Study the drawing (mm; zero at the part's minimum x, y, z) and answer. A direction names the side the tool comes from. Give positions to 0.01 mm unless a question says otherwise; leave off trailing zeros. Order: outer loops, then holes, each group sorted by start corner. A loop starts at its lowest first (then second) coordinate and runs counter-clockwise, first axis right, second up. Notation, with made-up numbers: (-32.75, 1.5) - (-10.75, 1.5) arc R29 cw to (-10.75, 37.5) - close; hole circle Ø11 at (27.5, -34.5). An arc over 180 degrees is marked (long way). Write each question's results on one line, items separated by ' | '. Start each with the question number.
1. Which of the six approach directions +Z, -Z, +X, -X, +Y, -Y give full straight-line access (tool end or side, diameter ignored) to the marked faces 4, 5 and 6?
2. Flat-ended cylindrical pins translate along their axes: pin 1 (2 mm diameter, centred on x = 10.5, y = 4, fed in from -Z); pin 2 (2 mm diameter, centred on x = 6.5, y = 7.5, fed in from +Z); pin 3 (1.5 mm diameter, centred on x = 4, z = 6.5, fed in from -Y). Find the tip coordinate at first contact, or state that the pin passes through.
3. Determine the mould class of the marked faces 1, 2 and 3 for opening direction X: released by +X, released by -X, zero draft, split by the parting line, or undercut.
4. Find the intervals of material crossed by L1, parallel to X at y = 1.5, z = 12; L2, parallel to Z at x = 1.5, y = 0.5; L3, parallel to Y at x = 3, z = 17.25, in increasing order.
5. Section B-B (z = 9.25) is taken. Give the vertices of the cut face in (x, y), and give its area (3 significant figures).
6. Section A-A (y = 3.75) is taken. Give the vertices of the cut face in (x, z), and give its area (3 significant figures).
7. Section C-C (x = 3.5) is taken. Give the vertices of the cut face in (y, z).
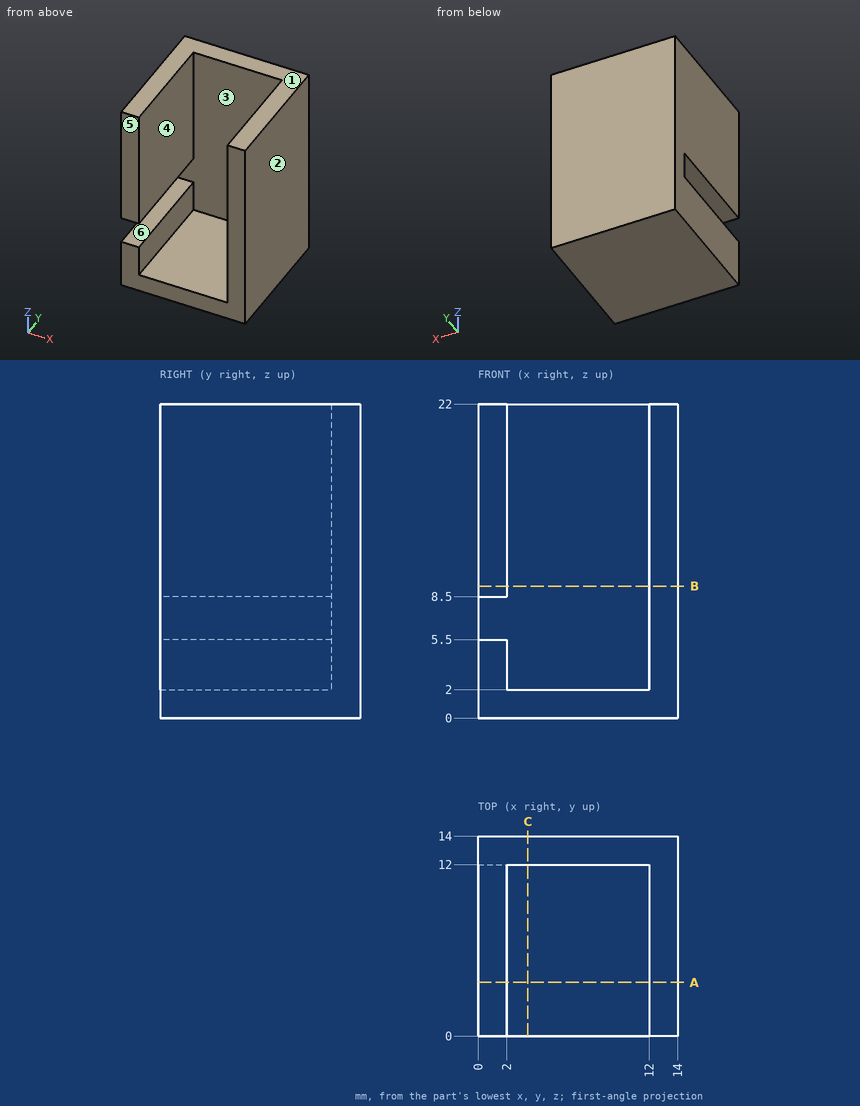
Reported:
1) face 4: +Z, -Y | face 5: +Z, -Z, +X, -X, -Y | face 6: -X, -Y
2) pin 1: z = 0 | pin 2: z = 2 | pin 3: y = 12
3) face 1: zero draft | face 2: released by +X | face 3: undercut
4) L1: 0 to 2, 12 to 14 | L2: 0 to 5.5, 8.5 to 22 | L3: 12 to 14
5) outline: (0, 0) - (2, 0) - (2, 12) - (12, 12) - (12, 0) - (14, 0) - (14, 14) - (0, 14) - close | area: 76.0 mm²
6) outline: (0, 0) - (14, 0) - (14, 22) - (12, 22) - (12, 2) - (2, 2) - (2, 5.5) - (0, 5.5) - close; (0, 8.5) - (2, 8.5) - (2, 22) - (0, 22) - close | area: 102 mm²
7) outline: (0, 0) - (14, 0) - (14, 22) - (12, 22) - (12, 2) - (0, 2) - close
